Could you check a few things on this model? Use its own coordinates, in mm. Round coordinates to 2 decimals unless told otherwise and drop trailing zeros. Loops run counter-clockwise (first coordinate to the right, second up) from the corner with the lowest first, then second, coordinate; pieces in that order, holes last. Notation, with made-up numbers: M 28,28 L 56,28 A10 cw 56,36 Z; hole C 27.25,23.25 d6. An arc over 180 degrees is marked long. One line per item, written item: value. Start each with the question number.
Q1. Imagine slicing it at B-B (x = 34.5). Please give me the cut outline in (y, z).
Q2. Imagine slicing it at A-A (y = -20). Please give me the cut outline in (x, z).
Q3. Please list where these lines run through material, in increasing order: line 1 along Z through (x, y) = (15.5, -20); line 2 along Z through (x, y) = (14, -27); line 3 along Y through (x, z) = (17.5, 37).
Q4. Thinking about a two-plate mould opening in Z: for faces 1 (the face through (20, -20, 0)), 2 (the face through (29, -40, 20)), 3 (the face through (20, -20, 40)), 4 (the face through (20.28, -10.46, 23)), which applies, released by +Z, released by -Z, zero draft, split by the parting line, or undercut?
Q5. I'm going to push flat-ended pins straight in: pin 1 Ø6 at (x, z) = (5.5, 29.5) entering from +Y; pin 2 Ø12 at (x, z) = (30, 11) entering from -Y; pin 3 Ø3 at (x, z) = (24.5, 23.5) entering from -Y. Where does each tip first touch, or does it pass through?
Q6. Imagine slicing it at C-C (z = 31.5). Please give me the cut outline in (x, y).
from build123d import *

# Parameters (mm, degrees)
F0_W     = 40
F0_H     = 40
F1_DEPTH = 40
F2_R     = 10
F3_DEPTH = 40.001


with BuildPart() as f1:
    # F0 (on Front) → F1 (new body)
    with BuildSketch(Plane.XZ):
        with Locations((20, 20)):
            Rectangle(F0_W, F0_H)
    extrude(amount=F1_DEPTH)

    # F2 (on face) → F3 (cut, through all)
    with BuildSketch(Plane.YZ.offset(40)):
        with Locations((-20, 20)):
            Circle(F2_R)
    extrude(amount=-F3_DEPTH, mode=Mode.SUBTRACT)

    # F4 (on face) → F5 (revolve)
    with BuildSketch(Plane.XZ.offset(40)):
        with BuildLine():
            ThreePointArc((11.028599, 20), (19.033267, 11.917013), (27.037935, 20))
            Line((27.037935, 20), (11.028599, 20))
        make_face()
    revolve(axis=Axis((19.033267, -40, 20), (-1, 0, 0)))


solid = f1.part
Report:
1. outline: M -40,0 L 0,0 L 0,40 L -40,40 Z; hole C -20,20 d20
2. outline: M 0,0 L 40,0 L 40,10 L 0,10 Z; M 0,30 L 40,30 L 40,40 L 0,40 Z
3. line 1: z = 0 to 10, 30 to 40
3. line 2: z = 0 to 12.86, 27.14 to 40
3. line 3: y = -40 to 0
4. face 1: released by -Z
4. face 2: zero draft
4. face 3: released by +Z
4. face 4: undercut
5. pin 1: stops at y = 0
5. pin 2: stops at y = -40
5. pin 3: stops at y = -46.34
6. outline: M 0,-40 L 40,-40 L 40,0 L 0,0 Z
